Study the drawing (mm; zero at the part's minimum x, y, z) and answer. A direction names the side the tool comes from. Coordinates: 2 decimals unless noted, no trailing zeros. Loops run counter-clockwise (first coordinate to the right, second up) from the corner with the lowest first, then second, coordinate; pieces in that order, holes last.
Q1. The mould has two halves that part along Y. Classify the marked faces 1, 2 and 3: pulls with the +Y half, pulls with the -Y half, needs draft (parallel to the pull), parting line crosses it, or undercut.
Q2. Flat-ended cylindrical pins translate along their axes: P1, Ø4, axis at y = 8.5, z = 11.5, coming from the +X side; P2, Ø5, axis at x = 17.5, z = 8.5, coming from the -Y side (1 decimal); P3, Ø3, axis at y = 11, z = 10, coming from the -X side. Find the tip coordinate at first contact, or state that the pin passes through.
Q3. Which of the six approach directions +Z, -Z, +X, -X, +Y, -Y give full straight-line access (tool end or side, diameter ignored) to the marked faces 4, 5, 6, 7 and 8?
Q4. Section D-D (y = 18) is taken. Give the vertices of the cut face in (x, z) (1 decimal), then the cut area to 3 significant figures.
Q5. Straight lines are drawn through the part: line 1 (Y direction, x = 11, z = 4); line 2 (X direction, y = 6.75, z = 5.5); line 3 (Z direction, x = 18, y = 5). For each, find the intervals that lie inside material, in ascending order.
Q6. Section C-C (x = 17.25) is taken. Give the vertices of the cut face in (y, z).
Q7. Section A-A (y = 11) is taken. Give the vertices of the cut face in (x, z).
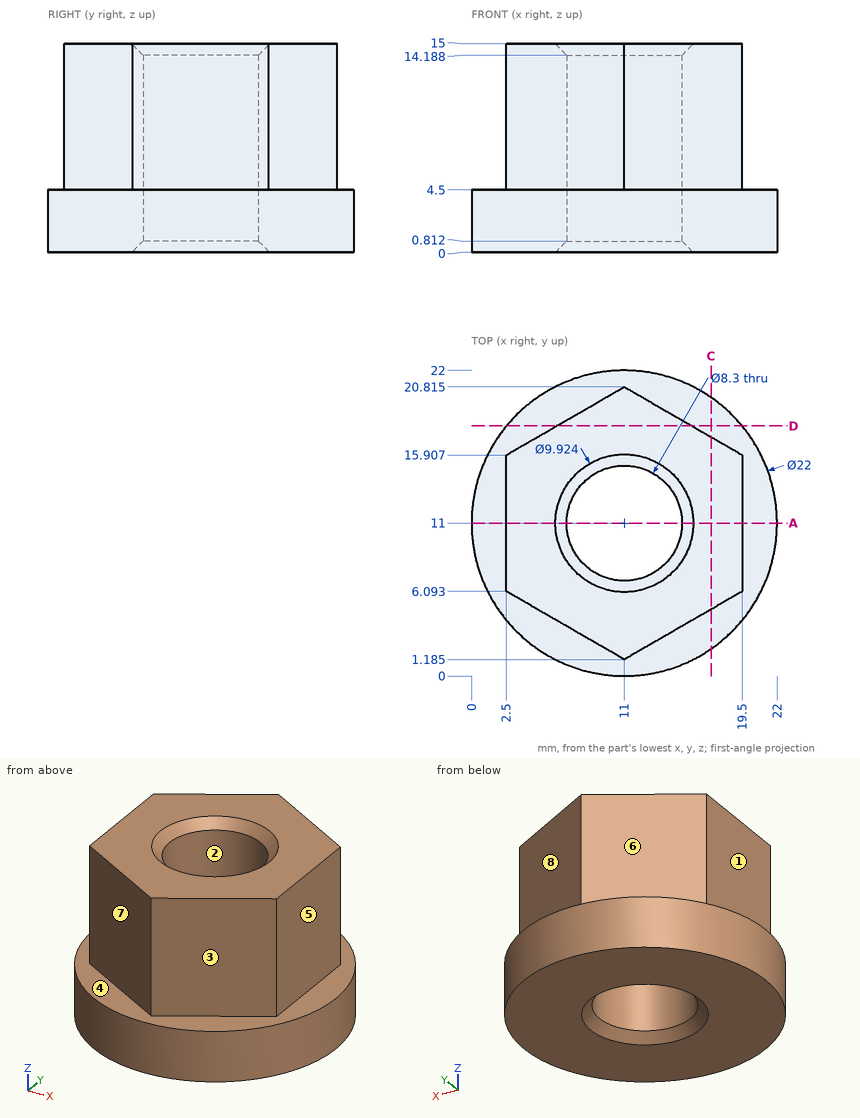
Numbers:
1. face 1: needs draft
1. face 2: undercut
1. face 3: pulls with the -Y half
2. P1: stops at x = 19.5
2. P2: stops at y = 3.5
2. P3: stops at x = 2.5
3. face 4: +Z
3. face 5: +Z, +X, +Y, -Y
3. face 6: +Z, -X, +Y
3. face 7: +Z, -X, -Y
3. face 8: +Z, +X, +Y
4. outline: (2.5, 0) - (19.5, 0) - (19.5, 4.5) - (15.9, 4.5) - (15.9, 15) - (6.1, 15) - (6.1, 4.5) - (2.5, 4.5) - close
4. area: 179 mm2
5. line 1: y = 0 to 6.85, 15.15 to 22
5. line 2: x = 2.5 to 19.5
5. line 3: z = 0 to 4.5
6. outline: (1.95, 0) - (20.05, 0) - (20.05, 4.5) - (17.21, 4.5) - (17.21, 15) - (4.79, 15) - (4.79, 4.5) - (1.95, 4.5) - close
7. outline: (0, 0) - (6.04, 0) - (6.85, 0.81) - (6.85, 14.19) - (6.04, 15) - (2.5, 15) - (2.5, 4.5) - (0, 4.5) - close; (15.15, 0.81) - (15.96, 0) - (22, 0) - (22, 4.5) - (19.5, 4.5) - (19.5, 15) - (15.96, 15) - (15.15, 14.19) - close
